```python
from build123d import *

# Parameters (mm, degrees)
SKETCH1_W           = 50
SKETCH1_H           = 80
BOSS_EXTRUDE5_DEPTH = 1.5
SKETCH4_R           = 1.3
BOSS_EXTRUDE6_DEPTH = 5
SKETCH6_R           = 2.15
SKETCH6_R_2         = 0.75
SKETCH6_W           = 1.2
SKETCH6_H           = 5.2
SKETCH6_W_2         = 2.5
SKETCH6_H_2         = 6
CUT_EXTRUDE1_DEPTH  = 10
FILLET1_R           = 2.5


with BuildPart() as part:
    # Sketch1 → Boss-Extrude5 (new body)
    with BuildSketch(Plane(origin=(0, 0, 0), x_dir=(0, 1, 0), z_dir=(0, 0, 1))):
        Rectangle(SKETCH1_W, SKETCH1_H)
    extrude(amount=BOSS_EXTRUDE5_DEPTH)

    # Sketch4 → Boss-Extrude6 (add)
    with BuildSketch(Plane(origin=(0, 0, 0), x_dir=(0, 1, 0), z_dir=(0, 0, 1))):
        with Locations(Location((-22.5, 37.5, 0), (0, 0, 90))):
            Circle(SKETCH4_R)
        with Locations(Location((0, 37.5, 0), (0, 0, 90))):
            Circle(SKETCH4_R)
        with Locations(Location((22.5, 37.5, 0), (0, 0, 90))):
            Circle(SKETCH4_R)
        with Locations(Location((-22.5, 0, 0), (0, 0, 90))):
            Circle(SKETCH4_R)
        with Locations(Location((22.5, 0, 0), (0, 0, 90))):
            Circle(SKETCH4_R)
        with Locations(Location((22.5, -37.5, 0), (0, 0, 90))):
            Circle(SKETCH4_R)
        with Locations(Location((0, -37.5, 0), (0, 0, 90))):
            Circle(SKETCH4_R)
        with Locations(Location((-22.5, -37.5, 0), (0, 0, 90))):
            Circle(SKETCH4_R)
    extrude(amount=BOSS_EXTRUDE6_DEPTH)

    # Sketch6 → Cut-Extrude1 (cut)
    with BuildSketch(Plane(origin=(0, 0, 0), x_dir=(0, 1, 0), z_dir=(0, 0, 1))):
        with Locations(Location((0, -20.25, 0), (0, 0, 90))):
            Circle(SKETCH6_R)
        with Locations(Location((-3.81, -17.71, 0), (0, 0, 90))):
            Circle(SKETCH6_R_2)
        with Locations(Location((2.54, -15.17, 0), (0, 0, 90))):
            Circle(SKETCH6_R_2)
        with Locations((7, 23.5)):
            Rectangle(SKETCH6_W, SKETCH6_H)
        with Locations((0, 23.5)):
            Rectangle(SKETCH6_W, SKETCH6_H)
        with Locations((-7, 23.5)):
            Rectangle(SKETCH6_W, SKETCH6_H)
        with Locations((0, 5.5)):
            Rectangle(SKETCH6_W, SKETCH6_H)
        with Locations((-7, 5.5)):
            Rectangle(SKETCH6_W, SKETCH6_H)
        with Locations((7, 5.5)):
            Rectangle(SKETCH6_W_2, SKETCH6_H_2)
    extrude(amount=CUT_EXTRUDE1_DEPTH, mode=Mode.SUBTRACT)

    # Fillet1
    fillet1_edges = [part.edges().sort_by_distance(p)[0] for p in [
        (-40, -25, 0.75),
        (-40, 25, 0.75),
        (40, -25, 0.75),
    ]]
    fillet(fillet1_edges, radius=FILLET1_R)


solid = part.part
```
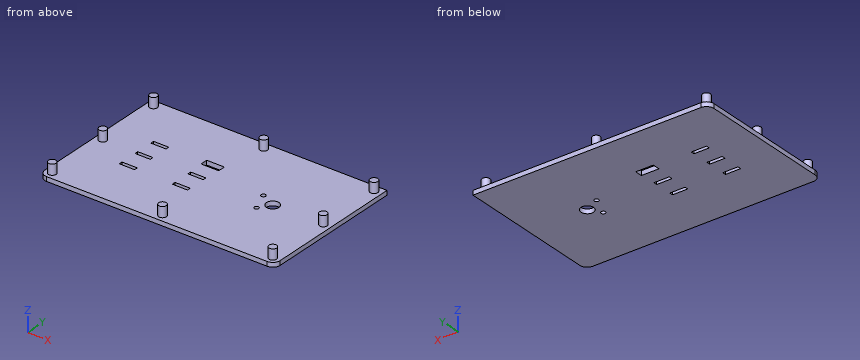
Check sheet for the modelled part. Datum: model origin and axes. Units: mm. Round coordinates to 2 decimals unless told otherwise and drop trailing zeros. Order: outer loops, then holes, each group sorted by start corner. A loop starts at its lowest first (then second) coordinate and runs counter-clockwise, first axis right, second up. Notation, with made-up numbers: (-34.75, -9.75) - (-24.75, -9.75) arc R16 ccw to (-24.75, 6.25) - close; hole circle Ø1 at (65.25, 89.25). An arc over 180 degrees is marked (long way). Write item = value, one per line.
Q1. Section check D-D (x = -11). Record the boundary of the cut face in (y, z), and give its area (3 significant figures).
Computed:
outline = (-25, 0) - (25, 0) - (25, 1.5) - (-25, 1.5) - close
area = 75.0 mm^2
Q2. Section check C-C (y = -15.5). Record the boundary of the cut face in (x, z).
Computed:
outline = (-40, 0) - (40, 0) - (40, 1.5) - (-40, 1.5) - close
Q3. Section check A-A (x = 20.25). Record the boundary of the cut face in (y, z), and give its area (4 significant figures).
Computed:
outline = (-25, 0) - (-2.15, 0) - (-2.15, 1.5) - (-25, 1.5) - close; (2.15, 0) - (25, 0) - (25, 1.5) - (2.15, 1.5) - close
area = 68.55 mm^2
Q4. Section check B-B (z = 0.75). State how many separate pieces and enclosed holes the cut face has, and give its area (3 significant figures).
Computed:
separate_pieces = 1
enclosed_holes = 9
area = 3,930 mm^2
Q5. Go/stop test with flat-tipped pins: pin 1 (1.2 mm diameter, centred on x = 17.71, y = -3.81, fed in from -Z); pin 2 (3 mm diameter, centred on x = -12, y = 4.5, fed in from +Z). Record where each tip stops, or that it passes through.
Computed:
pin_1 = through
pin_2 = 1.5
Q6. Thickness scan on line 1 along Y through (x, z) = (-22.5, 0.3); line 2 along Y through (x, z) = (17.71, 0.8); line 3 along Y through (x, z) = (15.17, 0.65). Record the ranges inside material, lowest first.
Computed:
line_1 = -25 to -7.6, -6.4 to -0.6, 0.6 to 6.4, 7.6 to 25
line_2 = -25 to -4.56, -3.06 to 25
line_3 = -25 to 1.79, 3.29 to 25
